```python
from build123d import *

# Parameters (mm, degrees)
BOSS_EXTRUDE1_DEPTH     = 18
BOSS_EXTRUDE1_2_DEPTH   = 18
CUT_EXTRUDE1_DEPTH      = 61.539243471
CUT_EXTRUDE1_DEPTH_BACK = 61.539243471
SKETCH3_R               = 3.1
CUT_EXTRUDE2_DEPTH      = 67.815043216
SKETCH5_R               = 3
CUT_EXTRUDE3_DEPTH      = 61.539243471
CHAMFER1_SIZE           = 1.5


with BuildPart() as part:
    # Sketch1 → Boss-Extrude1 (new, symmetric)
    with BuildSketch(Plane.XY):
        with BuildLine():
            Line((-13, 0), (-29, 0))
            Line((-29, 0), (-29, -1.5))
            Line((-29, -1.5), (-13, -1.5))
            ThreePointArc((-13, -1.5), (-11.939339828, -1.939339828), (-11.5, -3))
            Line((-11.5, -3), (-11.5, -50))
            Line((-11.5, -50), (-10, -50))
            Line((-10, -50), (-10, -3))
            ThreePointArc((-10, -3), (-10.878679656, -0.878679656), (-13, 0))
        make_face()
    extrude(amount=BOSS_EXTRUDE1_DEPTH, both=True)


with BuildPart() as body_2:
    # Sketch1 → Boss-Extrude1 2 (new, symmetric)
    with BuildSketch(Plane.XY):
        with BuildLine():
            Line((11.5, -50), (10, -50))
            Line((10, -50), (10, -3))
            ThreePointArc((10, -3), (10.878679656, -0.878679656), (13, 0))
            Line((13, 0), (29, 0))
            Line((29, 0), (29, -1.5))
            Line((29, -1.5), (13, -1.5))
            ThreePointArc((13, -1.5), (11.939339828, -1.939339828), (11.5, -3))
            Line((11.5, -3), (11.5, -50))
        make_face()
    extrude(amount=BOSS_EXTRUDE1_2_DEPTH, both=True)


with BuildPart() as cut_extrude1_tool:
    # Sketch2 → Cut-Extrude1 (new, two sides: drawn at the far end of the back side and taken through both)
    with BuildSketch(Plane(origin=(0, 0, 0), x_dir=(0, 0, -1), z_dir=(1, 0, 0)).offset(-CUT_EXTRUDE1_DEPTH_BACK)):
        Polygon((-18, -50), (-9, -50), (-18, -1.5), align=None)
        Polygon((9, -50), (18, -50), (18, -1.5), align=None)
    extrude(amount=CUT_EXTRUDE1_DEPTH + CUT_EXTRUDE1_DEPTH_BACK)


with BuildPart() as part_1:
    add(part.part)

    # Cut-Extrude1: cut by cut_extrude1_tool
    add(cut_extrude1_tool.part, mode=Mode.SUBTRACT)


with BuildPart() as body_2_1:
    add(body_2.part)

    # Cut-Extrude1: cut by cut_extrude1_tool
    add(cut_extrude1_tool.part, mode=Mode.SUBTRACT)


with BuildPart() as cut_extrude2_tool:
    # Sketch3 → Cut-Extrude2 (new, through all)
    with BuildSketch(Plane(origin=(11.5, 0, 0), x_dir=(0, 0, -1), z_dir=(1, 0, 0))):
        with Locations(Location((0, -40, 0), (0, 0, 90))):
            Circle(SKETCH3_R)
    extrude(amount=-CUT_EXTRUDE2_DEPTH)


with BuildPart() as part_2:
    add(part_1.part)

    # Cut-Extrude2: cut by cut_extrude2_tool
    add(cut_extrude2_tool.part, mode=Mode.SUBTRACT)



with BuildPart() as body_2_2:
    add(body_2_1.part)

    # Cut-Extrude2: cut by cut_extrude2_tool
    add(cut_extrude2_tool.part, mode=Mode.SUBTRACT)


with BuildPart() as part_3:
    add(part_2.part)

    add(body_2_2.part)  # Revolve1 merges body 2
    # Sketch4 → Revolve1 (revolve)
    with BuildSketch(Plane.XY, mode=Mode.PRIVATE) as revolve1_sk:
        Polygon((-10, -36.75), (10, -36.75), (10, -34.7), (9.3, -34), (-9.3, -34), (-10, -34.7), align=None)
    revolve(revolve1_sk.sketch.rotate(Axis((-10, -40, 0), (1, 0, 0)), 180), axis=Axis((-10, -40, 0), (1, 0, 0)))

    # Sketch5 → Cut-Extrude3 (cut, through all)
    with BuildSketch(Plane(origin=(0, 0, 0), x_dir=(1, 0, 0), z_dir=(0, 1, 0))):
        with Locations(Location((-20, 12.5, 0), (0, 0, 180))):
            Circle(SKETCH5_R)
        with Locations(Location((-20, -12.5, 0), (0, 0, 180))):
            Circle(SKETCH5_R)
        with Locations(Location((20, 12.5, 0), (0, 0, 180))):
            Circle(SKETCH5_R)
        with Locations(Location((20, -12.5, 0), (0, 0, 180))):
            Circle(SKETCH5_R)
    extrude(amount=-CUT_EXTRUDE3_DEPTH, mode=Mode.SUBTRACT)

    # Chamfer1
    chamfer1_edges = [part_3.edges().sort_by_distance(p)[0] for p in [
        (-29, -0.75, 18),
        (29, -0.75, -18),
        (29, -0.75, 18),
        (-29, -0.75, -18),
    ]]
    chamfer(chamfer1_edges, length=CHAMFER1_SIZE)


solid = part_3.part
```
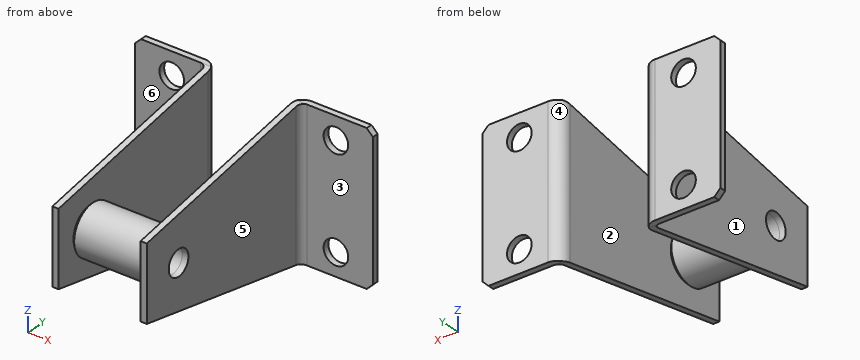
The listing builds one solid part. Answer for the finished solid, in the listing's coordinates (mm). Face numbers are marked on the shaded views. A direction names the side the tool comes from. Coordinates: 2 decimals unless noted, no trailing zeros. Write each loop counter-clockwise with the first axis right and the second up, starting at its lowest first coordinate (ties: lowest second). Pieces come first, ordered by that corner, then holes.
Q1. Section A-A, the plane z = -7 is taken. Write down the section's boundary in (x, y).
Returned:
outline: (-29, -1.5) - (-13, -1.5) arc R1.5 cw to (-11.5, -3) - (-11.5, -50) - (-10, -50) - (-10, -3) arc R3 ccw to (-13, 0) - (-29, 0) - close; (10, -50) - (11.5, -50) - (11.5, -3) arc R1.5 cw to (13, -1.5) - (29, -1.5) - (29, 0) - (13, 0) arc R3 ccw to (10, -3) - close
Q2. Which of the six approach directions +Z, -Z, +X, -X, +Y, -Y give full straight-line access (tool end or side, diameter ignored) to the marked faces 4, 5 and 6?
Returned:
face 4: +Z, -Z, +Y
face 5: +Z, -Z, +X, -Y
face 6: +Z, -Z, -X, -Y
Q3. Given P1, Ø1, axis at y = -8.5, z = -13, coming from the -X side; P2, Ø12, axis at x = -12.5, y = -32.5, coming from the -Z side; P3, Ø12, axis at x = 10.5, y = -12, coming from the +Z side, each flat-ended and moving along its own axis, determine where each tip first touches the part or whether it passes through.
Returned:
P1: stops at x = -11.5
P2: stops at z = -13.35
P3: stops at z = 17.16
Q4. Find the intervals of material crossed by line 1 along Z through (x, y) = (-20, -0.7); line 2 along X through (y, z) = (-46.5, -8); line 3 along Y through (x, z) = (26, 3.5), in increasing order.
Returned:
line 1: z = -18 to -15.5, -9.5 to 9.5, 15.5 to 18
line 2: x = -11.5 to -10, 10 to 11.5
line 3: y = -1.5 to 0
Q5. Section C-C, the plane y = -15.5 is taken. Write down the section's boundary in (x, z), then the cut area to 3 significant figures.
Returned:
outline: (-11.5, -15.4) - (-10, -15.4) - (-10, 15.4) - (-11.5, 15.4) - close; (10, -15.4) - (11.5, -15.4) - (11.5, 15.4) - (10, 15.4) - close
area: 92.4 mm2
Q6. Section D-D, the plane z = 12.5 is taken. Write down the section's boundary in (x, y), then the cut area to 3 significant figures.
Returned:
outline: (-29, -1.5) - (-23, -1.5) - (-23, 0) - (-29, 0) - close; (-17, -1.5) - (-13, -1.5) arc R1.5 cw to (-11.5, -3) - (-11.5, -31.14) - (-10, -31.14) - (-10, -3) arc R3 ccw to (-13, 0) - (-17, 0) - close; (10, -31.14) - (11.5, -31.14) - (11.5, -3) arc R1.5 cw to (13, -1.5) - (17, -1.5) - (17, 0) - (13, 0) arc R3 ccw to (10, -3) - close; (23, -1.5) - (29, -1.5) - (29, 0) - (23, 0) - close
area: 125 mm2
Q7. Section B-B, the plane x = -20 is taken. Write down the section's boundary in (y, z).
Returned:
outline: (-1.5, -18) - (0, -18) - (0, -15.5) - (-1.5, -15.5) - close; (-1.5, -9.5) - (0, -9.5) - (0, 9.5) - (-1.5, 9.5) - close; (-1.5, 15.5) - (0, 15.5) - (0, 18) - (-1.5, 18) - close
Q8. The mould has two halves that part along X. Classify the marked faces 1, 2 and 3: released by +X, released by -X, zero draft, split by the parting line, or undercut.
Returned:
face 1: released by -X
face 2: undercut
face 3: zero draft
